Model file for the job. Use its own axes, mm. Coordinates: 2 decimals unless noted, no trailing zeros. Write each loop counter-clockwise with the first axis right and the second up, starting at its lowest first coordinate (ties: lowest second). Pieces come first, ordered by that corner, then holes. Notation, with made-up numbers: (61.5, 1.25) -> (87.5, 1.25) arc R11 cw to (87.5, 19.25) -> close; hole circle Ø2 at (-11, 6.25). An arc over 180 degrees is marked (long way). Answer as a JSON object with one key per item and string values. Group by question number.
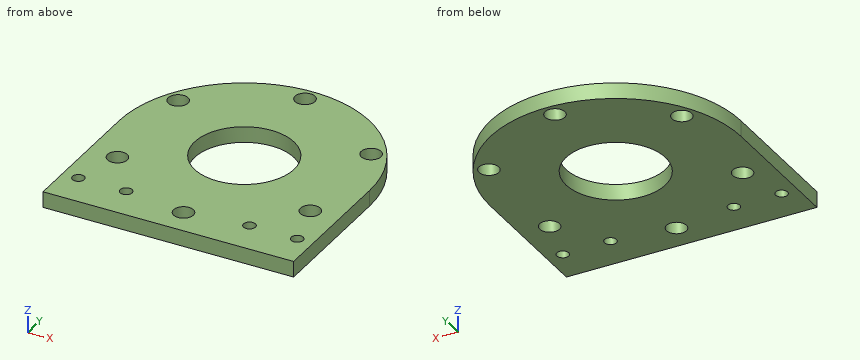
from build123d import *

# Parameters (mm, degrees)
SKETCH_1_R          = 31.5
EXTRUDE_1_DEPTH     = 4
SKETCH_2_R          = 12.5
SKETCH_2_R_2        = 2.5
CUT_EXTRUDE_1_DEPTH = 48.257274572
SKETCH_3_R          = 1.5
CUT_EXTRUDE_2_DEPTH = 48.257274572


with BuildPart() as part:
    # 草图1 → 凸台-拉伸1 (new body)
    with BuildSketch(Plane.XY):
        Circle(SKETCH_1_R)
        with BuildLine():
            ThreePointArc((31.5, 0), (0, -31.5), (-31.5, 0))
            Line((-31.5, 0), (-31.5, -35))
            Line((-31.5, -35), (31.5, -35))
            Line((31.5, -35), (31.5, 0))
        make_face()
    extrude(amount=EXTRUDE_1_DEPTH)

    # 草图2 → 切除-拉伸1 (cut, through all)
    with BuildSketch(Plane.XY.offset(4)):
        Circle(SKETCH_2_R)
        with Locations((0, 28)):
            Circle(SKETCH_2_R_2)
        with Locations((24.248711306, -14)):
            Circle(SKETCH_2_R_2)
        with Locations((-24.248711306, -14)):
            Circle(SKETCH_2_R_2)
        with Locations((0, -28)):
            Circle(SKETCH_2_R_2)
        with Locations((-24.248711306, 14)):
            Circle(SKETCH_2_R_2)
        with Locations((24.248711306, 14)):
            Circle(SKETCH_2_R_2)
    extrude(amount=-CUT_EXTRUDE_1_DEPTH, mode=Mode.SUBTRACT)

    # 草图3 → 切除-拉伸2 (cut, through all)
    with BuildSketch(Plane.XY.offset(4)):
        with Locations((-27.5, -26)):
            Circle(SKETCH_3_R)
        with Locations((-15.5, -26)):
            Circle(SKETCH_3_R)
        with Locations(Location((15.5, -26, 0), (0, 0, 180))):
            Circle(SKETCH_3_R)
        with Locations(Location((27.5, -26, 0), (0, 0, 180))):
            Circle(SKETCH_3_R)
    extrude(amount=-CUT_EXTRUDE_2_DEPTH, mode=Mode.SUBTRACT)


solid = part.part
(1) Cut at A-A on y = -29.5. List the corners of the cut face in (x, z).
(2) Cut at B-B on x = 0. List the corners of the cut face in (y, z), plus the area to 3 significant figures.
(3) Pin check, flat tip, straight feed: pin 1 (1 mm diameter, centred on y = 17.5, z = 3.5, fed in from -X). Stop position of the tip, or through.
(4) Cut at D-D on x = 15.5. List the corners of the cut face in (y, z).
(5) Cut at C-C on z = 2.9. Give the number of separate pieces and of enclosed holes in the cut face, plus the area to 3 significant figures.
(6) Wall check: probe 1 along Y at (x, z) = (0, 2.05); probe 2 along Y at (x, z) = (-25, 0.9); probe 3 along Y at (x, z) = (-24.5, 2.1). Give the ranges that are in metal, low to high.
Results found:
{
 "1": {"outline": "(-31.5, 0) -> (-2, 0) -> (-2, 4) -> (-31.5, 4) -> close; (2, 0) -> (31.5, 0) -> (31.5, 4) -> (2, 4) -> close"},
 "2": {"outline": "(-35, 0) -> (-30.5, 0) -> (-30.5, 4) -> (-35, 4) -> close; (-25.5, 0) -> (-12.5, 0) -> (-12.5, 4) -> (-25.5, 4) -> close; (12.5, 0) -> (25.5, 0) -> (25.5, 4) -> (12.5, 4) -> close; (30.5, 0) -> (31.5, 0) -> (31.5, 4) -> (30.5, 4) -> close", "area": "126 mm²"},
 "3": {"pin 1": "stops at x = -26.52"},
 "4": {"outline": "(-35, 0) -> (-27.5, 0) -> (-27.5, 4) -> (-35, 4) -> close; (-24.5, 0) -> (27.42, 0) -> (27.42, 4) -> (-24.5, 4) -> close"},
 "5": {"separate pieces": "1", "enclosed holes": "11", "area": "3,130 mm²"},
 "6": {"probe 1": "y = -35 to -30.5, -25.5 to -12.5, 12.5 to 25.5, 30.5 to 31.5", "probe 2": "y = -35 to -16.38, -11.62 to 11.62, 16.38 to 19.16", "probe 3": "y = -35 to -16.49, -11.51 to 11.51, 16.49 to 19.8"}
}
